Source: three-view drawing plus pictorial views. Frame: mm from the lowest corner of the part. A direction names the side the tool comes from. Coordinates: 2 decimals unless noted, no trailing zeros. Write each loop counter-clockwise with the first axis right and the second up, starting at its lowest first coordinate (ties: lowest second). Pieces come first, ordered by that corner, then holes. Notation, with made-up numbers: M -20.5,36 L 38.5,36 A19 ccw 38.5,50 Z; hole C 13,19.5 d5. An arc over 180 degrees is marked long. Write item = value, one per line. Start each with the question number.
Item 1: Section C-C on y = 12.5. Output: boundary loops of the cut face in (x, z).
Item 2: Reachability of the marked faces 1 and 2 from +Z, -Z, +X, -X, +Y, -Y: full face, straight path, thin tool, end or side. Return the list, or none.
Item 3: Ray query, L1, parallel to X at y = 1.7, z = 2.5; L2, parallel to Y at x = 8, z = 7; L3, parallel to X at y = 38, z = 7. Return the intervals inside material, ascending. Write a range as [from, to].
Item 4: Section A-A on x = 5. Output: boundary loops of the cut face in (y, z).
Item 5: Section B-B on z = 7.5. Output: boundary loops of the cut face in (x, y).
Item 6: First-contact query: pin 1 Ø5 at (y, z) = (32, 4.5) entering from -X; pin 2 Ø1.5 at (x, z) = (4.5, 5.5) entering from +Y. Flat tips, straight axial feed; report the tip coordinate or a pass-through.
Item 7: Section D-D on z = 2. Output: boundary loops of the cut face in (x, y), plus the area to 3 significant figures.
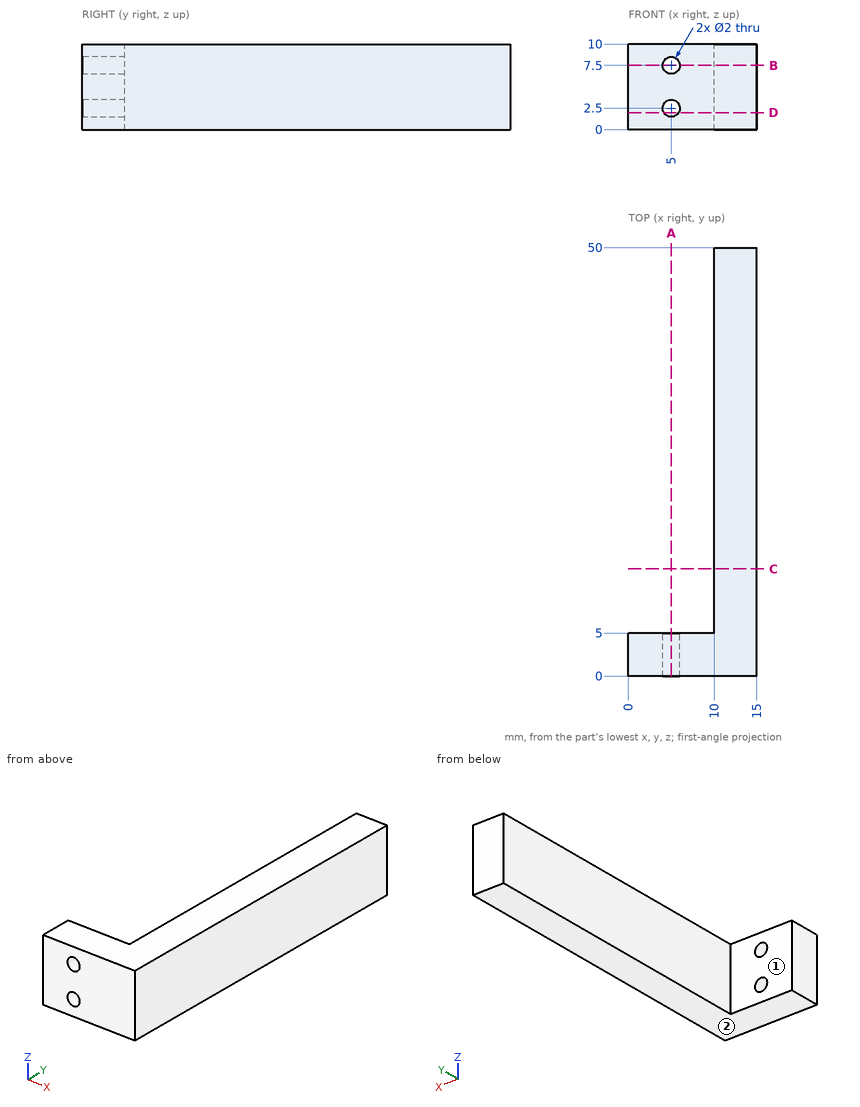
Responses:
q1.outline = M 10,0 L 15,0 L 15,10 L 10,10 Z
q2.face_1 = +Z, -Z, -X, +Y
q2.face_2 = -Z, +X, -X, +Y, -Y
q3.L1 = [0, 4], [6, 15]
q3.L2 = [0, 5]
q3.L3 = [10, 15]
q4.outline = M 0,0 L 5,0 L 5,1.5 L 0,1.5 Z; M 0,3.5 L 5,3.5 L 5,6.5 L 0,6.5 Z; M 0,8.5 L 5,8.5 L 5,10 L 0,10 Z
q5.outline = M 0,0 L 4,0 L 4,5 L 0,5 Z; M 6,0 L 15,0 L 15,50 L 10,50 L 10,5 L 6,5 Z
q6.pin_1 = 10
q6.pin_2 = 5
q7.outline = M 0,0 L 4.13,0 L 4.13,5 L 0,5 Z; M 5.87,0 L 15,0 L 15,50 L 10,50 L 10,5 L 5.87,5 Z
q7.area = 291 mm²
